Design review of the part shown in the three views and the two pictorial views. Dimensions are in mm from the part's minimum x, y and z. Coordinates: 2 decimals unless noted, no trailing zeros. Order: outer loops, then holes, each group sorted by start corner. A loop starts at its lowest first (then second) coordinate and runs counter-clockwise, first axis right, second up. Notation, with made-up numbers: (28.25, 38.5) -> (69.25, 38.5) arc R26 ccw to (69.25, 73.5) -> close; hole circle Ø4 at (-25.75, 5.5). An arc over 180 degrees is marked (long way). Write item = value, one per line. Start each with the question number.
1) Consider section B-B on x = 22. Give the boundary of the cut face in (y, z), and give its area (3 significant figures).
2) Consider section C-C on x = 32.5. Give the boundary of the cut face in (y, z) (1 decimal).
3) Insertion check: pin 1 Ø2 at (x, y) = (16, 70) entering from -Z; pin 2 Ø1 at (x, y) = (37.5, 63.5) entering from +Z. Each pin has a flat end and moves straight along its axis. Give the tip position at first contact, or say it passes through.
4) Consider section A-A on z = 1.5. Give the boundary of the cut face in (x, y) (1 decimal), and give its area (3 significant figures).
5) Wall thickness on probe 1 along Y at (x, z) = (52, 0.85); probe 2 along X at (y, z) = (59, 0.9); probe 3 along X at (y, z) = (64.5, 0.3): over which ranges is each line inside the solid? List them lowest first. Write a range as [from, to].
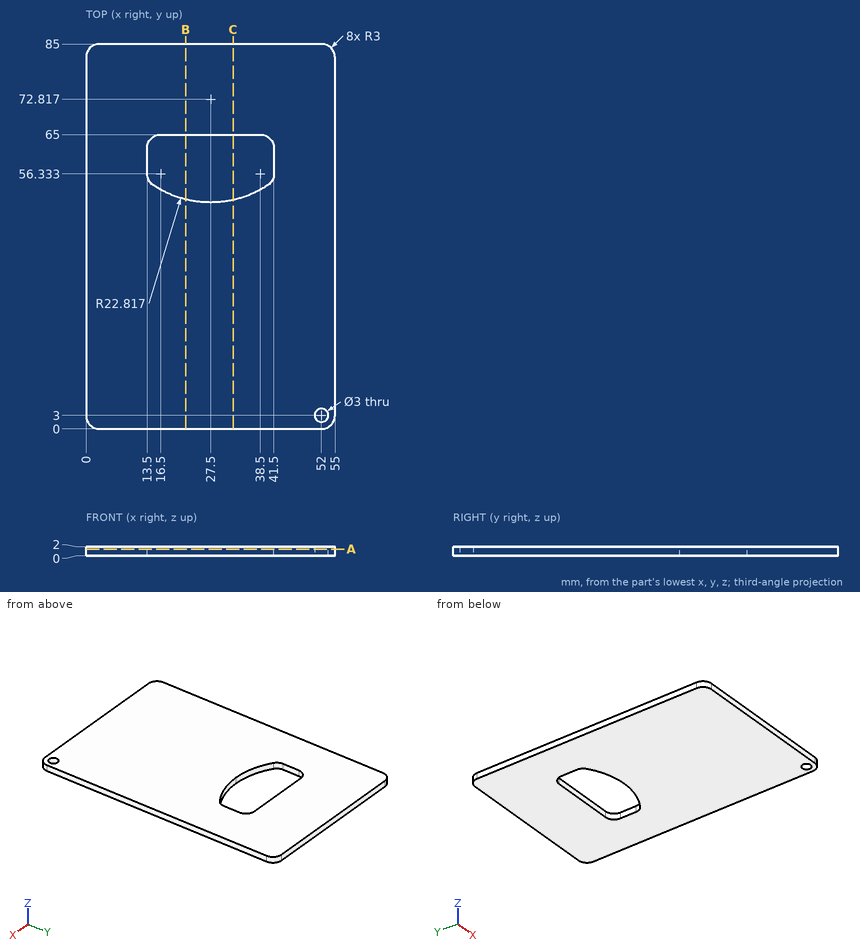
Answer sheet:
q1.outline = (0, 0) -> (50.67, 0) -> (50.67, 2) -> (0, 2) -> close; (65, 0) -> (85, 0) -> (85, 2) -> (65, 2) -> close
q1.area = 141 mm2
q2.outline = (0, 0) -> (50.6, 0) -> (50.6, 2) -> (0, 2) -> close; (65, 0) -> (85, 0) -> (85, 2) -> (65, 2) -> close
q3.pin_1 = 0
q3.pin_2 = through
q4.outline = (0, 3) arc R3 ccw to (3, 0) -> (52, 0) arc R3 ccw to (55, 3) -> (55, 82) arc R3 ccw to (52, 85) -> (3, 85) arc R3 ccw to (0, 82) -> close; hole (13.5, 56.3) arc R3 ccw to (14.8, 53.8) arc R22.8 ccw to (27.5, 50) arc R22.8 ccw to (40.2, 53.8) arc R3 ccw to (41.5, 56.3) -> (41.5, 62) arc R3 ccw to (38.5, 65) -> (16.5, 65) arc R3 ccw to (13.5, 62) -> close; hole circle Ø3 at (52, 3)
q4.area = 4,290 mm2
q5.probe_1 = [0, 1.5], [4.5, 85]
q5.probe_2 = [0, 13.5], [41.5, 55]
q5.probe_3 = [0, 14.84], [40.16, 55]
